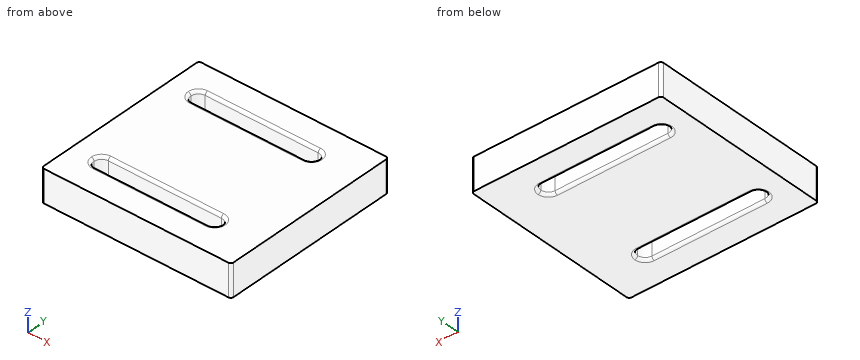
from build123d import *

# Parameters (mm, degrees)
F0_W     = 68
F0_H     = 65
F1_DEPTH = 11.6
F3_DEPTH = 25
F4_R     = 1


with BuildPart() as f1:
    # F0 (on Top) → F1 (new body)
    with BuildSketch(Plane.XY):
        with Locations((34, 32.5)):
            Rectangle(F0_W, F0_H)
    extrude(amount=F1_DEPTH)

    # F2 (on face) → F3 (cut)
    with BuildSketch(Plane.XY.offset(11.6)):
        with BuildLine():
            Line((51.25, 15.25), (10.75, 15.25))
            ThreePointArc((10.75, 15.25), (8.805456, 14.444544), (8, 12.5))
            ThreePointArc((8, 12.5), (8.805456, 10.555456), (10.75, 9.75))
            Line((10.75, 9.75), (51.25, 9.75))
            ThreePointArc((51.25, 9.75), (53.194544, 10.555456), (54, 12.5))
            ThreePointArc((54, 12.5), (53.194544, 14.444544), (51.25, 15.25))
        make_face()
        with BuildLine():
            Line((51.25, 55.25), (10.75, 55.25))
            ThreePointArc((10.75, 55.25), (8.805456, 54.444544), (8, 52.5))
            ThreePointArc((8, 52.5), (8.805456, 50.555456), (10.75, 49.75))
            Line((10.75, 49.75), (51.25, 49.75))
            ThreePointArc((51.25, 49.75), (53.194544, 50.555456), (54, 52.5))
            ThreePointArc((54, 52.5), (53.194544, 54.444544), (51.25, 55.25))
        make_face()
    extrude(amount=-F3_DEPTH, mode=Mode.SUBTRACT)

    # F4
    f4_edges = [f1.edges().sort_by_distance(p)[0] for p in [
        (31, 49.75, 0),
        (31, 9.75, 0),
        (31, 49.75, 11.6),
        (31, 15.25, 11.6),
        (68, 0, 5.8),
        (68, 65, 5.8),
        (0, 65, 5.8),
        (0, 0, 5.8),
    ]]
    fillet(f4_edges, radius=F4_R)


solid = f1.part
Design review of the part built by this model. Coordinates are the model's own, in mm. Round coordinates to 2 decimals unless told otherwise and drop trailing zeros. Write each loop counter-clockwise with the first axis right and the second up, starting at its lowest first coordinate (ties: lowest second). Pieces come first, ordered by that corner, then holes. Notation, with made-up numbers: M 36.5,-0.5 L 56.5,-0.5 A17 cw 56.5,18.5 Z; hole C 77.5,2 d3. An arc over 180 degrees is marked long. One line per item, written item: value. Start each with the question number.
1. Take a section at A-A on x = 26. State the section outline as (y, z) points.
2. Take a section at B-B on z = 6.5. State the section outline as (x, y) points, then the cut area to 3 significant figures.
3. Take a section at C-C on x = 9. State how many separate pieces and enclosed holes the cut face has, then the cut area to 3 significant figures.
4. To check wall thickness, follow probe 1 along Y at (x, z) = (35, 10.25); probe 2 along Y at (x, z) = (26.5, 0.5); probe 3 along X at (y, z) = (14, 5.75). State the ranges of each line that lie inside material, in increasing order. Write a range as from..to.
Computed:
1. outline: M 0,0 L 8.75,0 A1 ccw 9.75,1 L 9.75,10.6 A1 ccw 8.75,11.6 L 0,11.6 Z; M 15.25,1 A1 ccw 16.25,0 L 48.75,0 A1 ccw 49.75,1 L 49.75,10.6 A1 ccw 48.75,11.6 L 16.25,11.6 A1 ccw 15.25,10.6 Z; M 55.25,1 A1 ccw 56.25,0 L 65,0 L 65,11.6 L 56.25,11.6 A1 ccw 55.25,10.6 Z
2. outline: M 0,1 A1 ccw 1,0 L 67,0 A1 ccw 68,1 L 68,64 A1 ccw 67,65 L 1,65 A1 ccw 0,64 Z; hole M 8,12.5 A2.75 ccw 10.75,9.75 L 51.25,9.75 A2.75 ccw 54,12.5 A2.75 ccw 51.25,15.25 L 10.75,15.25 A2.75 ccw Z; hole M 8,52.5 A2.75 ccw 10.75,49.75 L 51.25,49.75 A2.75 ccw 54,52.5 A2.75 ccw 51.25,55.25 L 10.75,55.25 A2.75 ccw Z
2. area: 3,930 mm²
3. separate pieces: 3
3. enclosed holes: 0
3. area: 653 mm²
4. probe 1: y = 0..9.75, 15.25..49.75, 55.25..65
4. probe 2: y = 0..9.62, 15.38..49.62, 55.38..65
4. probe 3: x = 0..8.45, 53.55..68
